Design review of the part built by this model. Coordinates are the model's own, in mm. A direction names the side the tool comes from. Give positions to 0.01 mm unless a question says otherwise; leave off trailing zeros. Write each loop counter-clockwise with the first axis right and the second up, starting at its lowest first coordinate (ties: lowest second). Pieces come first, ordered by that corner, then holes. Notation, with made-up numbers: (-11, 40) -> (-6, 40) arc R16 cw to (-6, 68) -> close; hole circle Ø11 at (-19.5, 69). An arc over 180 degrees is marked (long way). Write each question's results on one line, items separated by ' | '. Start each with the question number.
(1) To check wall thickness, follow probe 1 along X at (y, z) = (1, -20.5); probe 2 along Z at (x, y) = (-96, 1.25); probe 3 along Z at (x, y) = (-159.5, 0.6). State the ranges of each line that lie inside material, in increasing order.
(2) Mouldability with a two-part tool opening along X and no side actions: class faces 3 (the face through (-71.655, 0.74, -62.115)), 4 (the face through (-2, 0, -19)), 5 (the face through (72.099, 0.74, -62.885)), 6 (the face through (162.15, 0.76, -91.99)) as released by +X, released by -X, zero draft, split by the parting line, or undercut.
(3) Take a section at A-A (x = -29). State the section outline as (y, z) points, plus the area to 3 significant figures.
(4) For faces 1 (the face through (65.49, 0.76, 7.85)), 2 (the face through (-161.99, 0.76, -92.15)), list the 3-axis set-ups (+Z, -Z, +X, -X, +Y, -Y) from which the entire face can be reached by the end or side of a thin tool; tool diameter is ignored.
(5) Take a section at B-B (y = 0.45). Count the separate pieces of the cut face and the enclosed holes in it, plus the area to 3 significant figures.
from build123d import *

# Parameters (mm, degrees)
BOSS_EXTRU_1_DEPTH      = 1.5
CONG_2_R                = 10
D_GAGEMENT_M31_D        = 3.4
ESQUISSE4_R             = 8.1
ESQUISSE4_W             = 13
ESQUISSE4_H             = 19.5
ENL_V_MAT_EXTRU_1_DEPTH = 191.400236344


with BuildPart() as part:
    # Esquisse1 → Boss.-Extru.1 (new body)
    with BuildSketch(Plane(origin=(0, 0, 0), x_dir=(1, 0, 0), z_dir=(0, 1, 0))):
        Polygon((-165, -30), (-68.5, -30), (-68.5, -5), (68.5, -5), (68.5, -30), (165, -30), (165, 90), (165, 95), (90.641016151, 95), (53.113248654, 30), (-53.113248654, 30), (-90.641016151, 95), (-165, 95), (-165, 90), align=None)
    extrude(amount=BOSS_EXTRU_1_DEPTH)

    # Congé2
    cong_2_edges = [part.edges().sort_by_distance(p)[0] for p in [
        (68.5, 0.75, 30),
        (68.5, 0.75, 5),
        (-68.5, 0.75, 5),
        (-68.5, 0.75, 30),
        (-165, 0.75, 30),
        (-165, 0.75, -95),
        (-90.641016151, 0.75, -95),
        (-53.113248654, 0.75, -30),
        (53.113248654, 0.75, -30),
        (90.641016151, 0.75, -95),
        (165, 0.75, -95),
        (165, 0.75, 30),
    ]]
    fillet(cong_2_edges, radius=CONG_2_R)

    # Dégagement M31 (through all)
    with Locations(Plane(origin=(0, 1.5, 0), x_dir=(1, 0, 0), z_dir=(0, 1, 0))):
        with Locations((-75.5, -16.5), (-75.5, 3.5), (75.5, -16.5), (75.5, 3.5), (-145.5, -24.5), (-159.5, -10.5), (-159.5, 70.5), (-145.5, 84.5), (145.5, -24.5), (159.5, -10.5), (145.5, 84.5), (159.5, 70.5), (-43.58, 20.5), (43.58, 20.5), (-106.53, 84.5), (106.53, 84.5)):
            Hole(D_GAGEMENT_M31_D / 2)

    # Esquisse4 → Enlèv. mat.-Extru.1 (cut, through all)
    with BuildSketch(Plane(origin=(0, 1.5, 0), x_dir=(1, 0, 0), z_dir=(0, 1, 0))):
        with Locations(Location((-125, -13.9, 0), (0, 0, 270))):
            Circle(ESQUISSE4_R)
        with Locations((-95, -12.25)):
            Rectangle(ESQUISSE4_W, ESQUISSE4_H)
    extrude(amount=-ENL_V_MAT_EXTRU_1_DEPTH, mode=Mode.SUBTRACT)


solid = part.part
Report:
1) probe 1: -165 to -45.28, -41.88 to 41.88, 45.28 to 165 | probe 2: -94.99 to 2.5, 22 to 30 | probe 3: -93.93 to -72.2, -68.8 to 8.8, 12.2 to 28.93
2) face 3: undercut | face 4: zero draft | face 5: undercut | face 6: released by +X
3) outline: (0, -30) -> (1.5, -30) -> (1.5, 5) -> (0, 5) -> close | area: 52.5 mm2
4) face 1: +Z, +Y, -Y | face 2: -Z, -X, +Y, -Y
5) separate pieces: 1 | enclosed holes: 18 | area: 27,800 mm2
